Geometry check sheet. Reference: the model listing, model coordinates, mm. Face numbers are marked on the shaded views. Coordinates: 2 decimals unless noted, no trailing zeros. Loops run counter-clockwise (first coordinate to the right, second up) from the corner with the lowest first, then second, coordinate; pieces in that order, holes last. Notation, with made-up numbers: (-28.5, 19) - (8.5, 19) arc R19 cw to (8.5, 35) - close; hole circle Ø10 at (70, 70.25). An arc over 180 degrees is marked (long way). One line per item, written item: value.
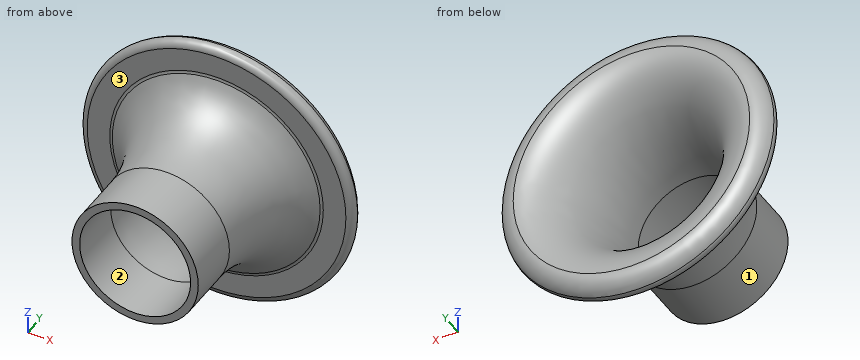
from build123d import *


with BuildPart() as f1:
    # F0 (on Top) → F1 (revolve)
    with BuildSketch(Plane.XY):
        with BuildLine():
            ThreePointArc((59.1817405743, 40.9936836903), (61.8067292629, 42.3826099559), (62.1350781175, 45.3341974637))
            ThreePointArc((62.1350781175, 45.3341974637), (58.9601205576, 49.303969233), (54.102, 50.8))
            add(Edge.make_bspline(
                [(54.102, 50.8), (25.4, 50.8), (25.4, 0)],
                knots=[0, 0, 0, 1.5707963268, 1.5707963268, 1.5707963268], degree=2, weights=[1, 0.7071067812, 1]))
            Line((25.4, 0), (25.4, -25.4))
            Line((25.4, -25.4), (28.8925, -25.4))
            Line((28.8925, -25.4), (28.8925, 0))
            add(Edge.make_bspline(
                [(47.5468117709, 40.7135982273), (28.8925, 32.3116489326), (28.8925, 0)],
                knots=[0.2630517082, 0.2630517082, 0.2630517082, 1.5707963268, 1.5707963268, 1.5707963268], degree=2, weights=[1, 0.7937343669, 1]))
            ThreePointArc((47.5468117709, 40.7135982273), (48.1838785423, 40.922872687), (48.8506886146, 40.9936836903))
            Line((48.8506886146, 40.9936836903), (59.1817405743, 40.9936836903))
        make_face()
    revolve(axis=Axis((0, 35.1700206795, 0), (0, 1, 0)))


solid = f1.part
(1) Cross-section at A-A on y = -16.5. Record the cut outline in (x, z) (1 decimal), and give its area (3 significant figures).
Reply:
outline: circle Ø57.8 at (0, 0); hole circle Ø50.8 at (0, 0)
area: 596 mm2
(2) Material ranges on probe 1 along Z at (x, y) = (0, -10.75); probe 2 along Y at (x, z) = (-32, -44.5), recorded low to high. Write a range as from..to.
Reply:
probe 1: -28.89..-25.4, 25.4..28.89
probe 2: 40.99..50.77
(3) Go/stop test with flat-tipped pins: pin 1 Ø10 at (y, z) = (26.5, -24.5) entering from +X; pin 2 Ø4 at (x, z) = (42, 46.5) entering from +Y; pin 3 Ø1 at (x, y) = (-18, 29) entering from +Z. Record where each tip stops, or that it passes through.
Reply:
pin 1: x = 29.77
pin 2: y = 47.78
pin 3: z = 31.39
(4) Release check for a two-part mould opening along Z. For the marked faces 1, 2 and 3 record: pulls with the +Z half, pulls with the -Z half, needs draft (parallel to the pull), parting line crosses it, or undercut.
Reply:
face 1: parting line crosses it
face 2: undercut
face 3: needs draft
